Solid Edge part; units mm, degrees
sketch "Sketch1" plane through (0, 0, 0) normal (0, 0, 1) x (1, 0, 0)
  line L0 (-57.5, -12.25) -> (57.5, -12.25)
  line L1 (57.5, -12.25) -> (57.5, 12.25)
  line L2 (57.5, 12.25) -> (-57.5, 12.25)
  line L3 (-57.5, 12.25) -> (-57.5, -12.25)
extrude "Protrusion1" add sketch "Sketch1" against normal blind 40
sketch "Sketch2" plane through (0, -12.25, -20) normal (0, -1, 0) x (1, 0, 0)
  line L0 (-57.5, 20) -> (-12.5, 20)
  line L1 (-12.5, 20) -> (-12.5, 13.5)
  line L2 (-12.5, 13.5) -> (-57.5, 13.5)
  line L3 (-57.5, 13.5) -> (-57.5, 20)
  line L4 (-57.5, -20) -> (-12.5, -20)
  line L5 (-12.5, -20) -> (-12.5, -13.5)
  line L6 (-12.5, -13.5) -> (-57.5, -13.5)
  line L7 (-57.5, -13.5) -> (-57.5, -20)
extrude "ExtrudedCutout_1" cut sketch "Sketch2" against normal blind 24.5
sketch "Sketch3" plane through (0, -12.25, -20) normal (0, -1, 0) x (1, 0, 0)
  line L0 (57.5, 20) -> (-12.5, 20)
  line L1 (-12.5, 20) -> (-12.5, 10)
  line L2 (-12.5, 10) -> (57.5, 10)
  line L3 (57.5, 10) -> (57.5, 20)
  line L4 (57.5, -20) -> (-12.5, -20)
  line L5 (-12.5, -20) -> (-12.5, -10)
  line L6 (-12.5, -10) -> (57.5, -10)
  line L7 (57.5, -10) -> (57.5, -20)
extrude "ExtrudedCutout_2" cut sketch "Sketch3" against normal blind 14.5
sketch "Sketch4" plane through (0, -12.25, -20) normal (0, -1, 0) x (1, 0, 0)
  line L0 (-47.5, 13.5) -> (-47.5, 12.5)
  line L1 (-47.5, 12.5) -> (-27.5, 12.5)
  line L2 (-27.5, 12.5) -> (-27.5, 13.5)
  line L3 (-27.5, 13.5) -> (-47.5, 13.5)
  line L4 (-47.5, -13.5) -> (-47.5, -12.5)
  line L5 (-47.5, -12.5) -> (-27.5, -12.5)
  line L6 (-27.5, -12.5) -> (-27.5, -13.5)
  line L7 (-27.5, -13.5) -> (-47.5, -13.5)
extrude "ExtrudedCutout_3" cut sketch "Sketch4" against normal blind 24.5
sketch "Sketch5" plane through (-20, 0, -6.5) normal (0, 0, 1) x (1, 0, 0)
  line L0 (-37.5, 12.25) -> (-37.5, 6.25)
  line L1 (-37.5, 6.25) -> (7.5, 6.25)
  line L2 (7.5, 6.25) -> (7.5, 12.25)
  line L3 (7.5, 12.25) -> (-37.5, 12.25)
  line L4 (-37.5, -12.25) -> (-37.5, -10.75)
  line L5 (-37.5, -10.75) -> (7.5, -10.75)
  line L6 (7.5, -10.75) -> (7.5, -12.25)
  line L7 (7.5, -12.25) -> (-37.5, -12.25)
extrude "ExtrudedCutout_4" cut sketch "Sketch5" against normal blind 40
sketch "Sketch6" plane through (22.5, -12.25, -20) normal (0, -1, 0) x (0, 0, 1)
  line L0 (20, -35) -> (20, -13.6)
  line L1 (20, -13.6) -> (10, -13.6)
  line L2 (10, -13.6) -> (10, -35)
  line L3 (10, -35) -> (20, -35)
extrude "ExtrudedCutout_5" cut sketch "Sketch6" against normal blind 34.9193
sketch "Sketch7" plane through (22.5, 2.25, -35) normal (0, -1, 0) x (1, 0, 0)
  line L0 (35, 5) -> (13.6, 5)
  line L1 (13.6, 5) -> (13.6, -5)
  line L2 (13.6, -5) -> (35, -5)
  line L3 (35, -5) -> (35, 5)
extrude "ExtrudedCutout_6" cut sketch "Sketch7" against normal blind 93.3643
sketch "Sketch8" plane through (22.5, -12.25, -20) normal (0, -1, 0) x (1, 0, 0)
  line L0 (-15, 20) -> (13.6, 10)
  line L1 (13.6, 10) -> (13.6, 20)
  line L2 (13.6, 20) -> (-15, 20)
extrude "ExtrudedCutout_7" cut sketch "Sketch8" against normal blind 164.1639
sketch "Sketch9" plane through (0, 0, 0) normal (0, 0, 1) x (1, 0, 0)
  line L0 (18.5, 2.25) -> (36.1, 12.25)
  line L1 (36.1, 12.25) -> (36.1, 2.25)
  line L2 (36.1, 2.25) -> (18.5, 2.25)
extrude "ExtrudedCutout_10" cut sketch "Sketch9" against normal blind 10
sketch "Sketch10" plane through (11.8, 7.25, -40) normal (0, 0, -1) x (0, -1, 0)
  line L0 (5, -6.7) -> (-5, -24.3)
  line L1 (-5, -24.3) -> (5, -24.3)
  line L2 (5, -24.3) -> (5, -6.7)
extrude "ExtrudedCutout_11" cut sketch "Sketch10" against normal blind 10
sketch "Sketch11" plane through (22.5, 12.25, -20) normal (0, 1, 0) x (0, 0, -1)
  line L0 (20, 15) -> (10, -13.6)
  line L1 (10, -13.6) -> (20, -13.6)
  line L2 (20, -13.6) -> (20, 15)
extrude "ExtrudedCutout_12" cut sketch "Sketch11" against normal blind 63.6065
sketch "Sketch12" plane through (0, 0, 0) normal (0, 0, 1) x (1, 0, 0)
  line L0 (57.5, 12.25) -> (57.5, 0)
  arc A0 (21.8, 12.25) -> (57.5, 0) centre (21.8, -45.895) cw
  line L1 (57.5, 12.25) -> (21.8, 12.25)
extrude "ExtrudedCutout_15" cut sketch "Sketch12" against normal blind 40
chamfer "Chamfer_1" distance 3 angle 45 4 edges at (-57.5, -2.25, -6.5) (-57.5, 6.25, -20) (-57.5, -2.25, -33.5) (-57.5, -10.75, -20)
Can you work these out from the model? Positions are in its coordinate system, mm. A direction names the side the tool comes from. Coordinates: 2 decimals unless noted, no trailing zeros. Loops run counter-clockwise (first coordinate to the right, second up) from the corner with the lowest first, then second, coordinate; pieces in that order, holes last. Notation, with made-up numbers: (48, 59.25) - (91, 59.25) arc R6 ccw to (91, 70.25) - close; hole circle Ø11 at (44, -2). An arc over 180 degrees is marked (long way). Answer as a JSON object with one key per item and string values. Group by question number.
Item 1: If we section it at B-B (z = -28): List the corners of the cut face in (x, y) for me (3 decimals).
Item 2: If we section it at C-C (x = -1): List the corners of the cut face in (y, z) for me.
Item 3: If we section it at D-D (y = -9): List the corners of the cut face in (x, z) for me.
Item 4: For pin 1 (11.5 mm diameter, centred on x = 27.5, y = 1, fed in from -Z); pin 2 (11 mm diameter, centred on x = 10, z = -36.5, fed in from -Y); pin 3 (13.5 mm diameter, centred on x = -41.5, y = -5, fed in from +Z), each with a flat end and sliding along its axis, tell me the tip position at first contact or that it passes through.
Item 5: If we mould it in two halves opening along X, with no side actions, what happens to faces 1 (the face through (-38, -2, -32.5)), 2 (the face through (17.57, 8.43, -36.48)), 3 (the face through (-34, -10.75, -20)), 4 (the face through (-56, -2, -32))? For each: released by +X, released by -X, zero draft, split by the parting line, or undercut.
Item 6: If I drill on L1, parallel to Y at x = -38, z = -22.5; L2, parallel to Z at x = -43, y = 5.5; L3, parallel to Y at x = 6.5, z = -37.5, over which ranges is the centre line in solid material (lowest first)? Write a range as from..to.
Item 7: If we section it at A-A (y = -1): List the corners of the cut face in (x, z) for me, plus the area to 3 significant figures.
Item 8: On a 3-axis mill with a long thin cutter (end or side, diameter ignored), from which of +Z, -Z, +X, -X, +Y, -Y can I reach the whole of each face in a straight line? I mean faces 5 (the face through (-34, 6.25, -20)), 6 (the face through (-51, -2, -6.5)), 7 (the face through (-20, -2, -33.5)), 8 (the face through (22, -3, -10)), 9 (the face through (-56.02, -9.23, -20.19)). Say none if no direction works.
Returned:
{
 "1": {"outline": "(-57.5, -7.75) - (-54.5, -10.75) - (-12.5, -10.75) - (-12.5, -12.25) - (57.5, -12.25) - (57.5, 0) arc R58.145 ccw to (21.8, 12.25) - (-12.5, 12.25) - (-12.5, 6.25) - (-54.5, 6.25) - (-57.5, 3.25) - close"},
 "2": {"outline": "(-12.25, -30) - (2.25, -30) - (2.25, -40) - (12.25, -40) - (12.25, 0) - (2.25, 0) - (2.25, -10) - (-12.25, -10) - close"},
 "3": {"outline": "(-56.25, -31.75) - (-54.5, -33.5) - (-47.5, -33.5) - (-47.5, -32.5) - (-27.5, -32.5) - (-27.5, -33.5) - (-12.5, -33.5) - (-12.5, -30) - (57.5, -30) - (57.5, -10) - (-12.5, -10) - (-12.5, -6.5) - (-27.5, -6.5) - (-27.5, -7.5) - (-47.5, -7.5) - (-47.5, -6.5) - (-54.5, -6.5) - (-56.25, -8.25) - close"},
 "4": {"pin 1": "stops at z = -34.44", "pin 2": "stops at y = 2.25", "pin 3": "stops at z = -6.5"},
 "5": {"face 1": "undercut", "face 2": "released by +X", "face 3": "zero draft", "face 4": "released by -X"},
 "6": {"L1": "y = -10.75..6.25", "L2": "z = -32.5..-7.5", "L3": "y = 2.25..12.25"},
 "7": {"outline": "(-57.5, -30.5) - (-54.5, -33.5) - (-47.5, -33.5) - (-47.5, -32.5) - (-27.5, -32.5) - (-27.5, -33.5) - (-12.5, -33.5) - (-12.5, -30) - (57.5, -30) - (57.5, -10) - (-12.5, -10) - (-12.5, -6.5) - (-27.5, -6.5) - (-27.5, -7.5) - (-47.5, -7.5) - (-47.5, -6.5) - (-54.5, -6.5) - (-57.5, -9.5) - close", "area": "2,570 mm²"},
 "8": {"face 5": "+Z, -Z, -X, +Y", "face 6": "+Z, -X, +Y, -Y", "face 7": "-Z, -X, +Y, -Y", "face 8": "+Z, +X, -Y", "face 9": "+Z, -Z, -X, -Y"}
}
